from build123d import *

# Parameters (mm, degrees)
F0_W      = 57.15
F0_H      = 38.1
F1_DEPTH  = 58.42
F2_W      = 25.4
F2_H      = 25.4
F3_DEPTH  = 25.4
F4_W      = 50.8
F4_H      = 25.4
F5_DEPTH  = 50.8
F6_W      = 20.32
F6_H      = 20.32
F7_DEPTH  = 81.28
F8_W      = 22.86
F8_H      = 12.7
F9_DEPTH  = 25.4
F10_W     = 6.35
F10_H     = 6.35
F10_W_2   = 15.24
F10_H_2   = 5.08
F11_DEPTH = 12.7
F12_W     = 25.4
F12_H     = 9.817438
F13_DEPTH = 12.7
F14_W     = 19.21422
F14_H     = 50.8
F15_DEPTH = 6.35


with BuildPart() as f1:
    # F0 (on Top) → F1 (new body)
    with BuildSketch(Plane.XY):
        Rectangle(F0_W, F0_H)
    extrude(amount=F1_DEPTH)

    # F2 (on face) → F3 (join)
    with BuildSketch(Plane.XY.offset(58.42)):
        Rectangle(F2_W, F2_H)
    extrude(amount=F3_DEPTH)

    # F4 (on face) → F5 (cut)
    with BuildSketch(Plane.XY):
        Rectangle(F4_W, F4_H)
    extrude(amount=F5_DEPTH, mode=Mode.SUBTRACT)

    # F6 (on face) → F7 (cut)
    with BuildSketch(Plane.XY):
        Rectangle(F6_W, F6_H)
    extrude(amount=F7_DEPTH, mode=Mode.SUBTRACT)

    # F8 (on face) → F9 (cut)
    with BuildSketch(Plane(origin=(-28.575, 0, 0), x_dir=(0, -1, 0), z_dir=(-1, 0, 0))):
        with Locations((0, 31.75)):
            Rectangle(F8_W, F8_H)
    extrude(amount=-F9_DEPTH, mode=Mode.SUBTRACT)

    # F10 (on face) → F11 (cut)
    with BuildSketch(Plane(origin=(0, 12.7, 0), x_dir=(-1, 0, 0), z_dir=(0, 1, 0))):
        with Locations((-5.08, 74.295)):
            Rectangle(F10_W, F10_H)
        with Locations((5.08, 74.295)):
            Rectangle(F10_W, F10_H)
        with Locations((0, 63.942472)):
            Rectangle(F10_W_2, F10_H_2)
    extrude(amount=-F11_DEPTH, mode=Mode.SUBTRACT)

    # F12 (on face) → F13 (cut)
    with BuildSketch(Plane(origin=(0, 19.05, 0), x_dir=(-1, 0, 0), z_dir=(0, 1, 0))):
        with Locations((0, 15.411281)):
            Rectangle(F12_W, F12_H)
    extrude(amount=-F13_DEPTH, mode=Mode.SUBTRACT)

    # F14 (on face) → F15 (join)
    with BuildSketch(Plane.YZ.offset(28.575)):
        with Locations((0, 25.4)):
            Rectangle(F14_W, F14_H)
    extrude(amount=F15_DEPTH)


solid = f1.part
Design review of the part built by this model. Coordinates are the model's own, in mm. A direction names the side the tool comes from. Give positions to 0.01 mm unless a question says otherwise; leave off trailing zeros. Write each loop counter-clockwise with the first axis right and the second up, starting at its lowest first coordinate (ties: lowest second). Pieces come first, ordered by that corner, then holes. Notation, with made-up numbers: M 7.25,-25 L 60.25,-25 A8 cw 60.25,-15 Z; hole C 88.25,89 d6. An arc over 180 degrees is marked long. Answer as a JSON object with one key per item and string values. Group by question number.
1) Tool access review of faces 1 (the face through (-27, 0, 38.1)), 2 (the face through (12.7, 16, 15)), 3 (the face through (0, 12.7, 71)), 4 (the face through (0, 12.7, 25)): name each direction out of +Z, -Z, +X, -X, +Y, -Y from which nothing blocks a thin tool from reaching the whole face with its end or side.
2) Mouldability with a two-part tool opening along X and no side actions: class faces 5 (the face through (0, -12.7, 25)), 6 (the face through (-28.575, 0, 22)), 7 (the face through (-27, -11.43, 32)) as released by +X, released by -X, zero draft, split by the parting line, or undercut.
3) We need section A-A (y = 17). Give the boundary of the cut face in (x, z) (3 decimals).
4) Clearance check with flat-ended pins moving along their axes: pin 1 Ø1.3 at (y, z) = (12, 74) entering from -X; pin 2 Ø1.9 at (x, y) = (33, -1.5) entering from +Z; pin 3 Ø3 at (x, z) = (-2.5, 70) entering from -Y. State where each tip first meets the part, or that it passes through.
5) We need section D-D (x = 22). Give the boundary of the cut face in (y, z), and give its area (3 significant figures).
6) For line 1 along Y through (x, z) = (-16, 50); line 2 along X through (y, z) = (-3, 52) (3 decimals); line 3 along X through (y, z) = (10, 14) (3 decimals), list the stretches that pass through material, from the lowest coordinate up.
7) We need section B-B (y = -7.5). Give the boundary of the cut face in (x, z) (3 decimals).
8) We need section C-C (z = 47). Give the boundary of the cut face in (x, y) (3 decimals).
Answer key:
{
 "1": {"face 1": "-X", "face 2": "+Y", "face 3": "+Z, +X, -X, +Y", "face 4": "-Z"},
 "2": {"face 5": "undercut", "face 6": "released by -X", "face 7": "zero draft"},
 "3": {"outline": "M -28.575,0 L 28.575,0 L 28.575,58.42 L -28.575,58.42 Z; hole M -12.7,10.503 L 12.7,10.503 L 12.7,20.32 L -12.7,20.32 Z"},
 "4": {"pin 1": "stops at x = -12.7", "pin 2": "stops at z = 50.8", "pin 3": "stops at y = -12.7"},
 "5": {"outline": "M -19.05,0 L -12.7,0 L -12.7,50.8 L 12.7,50.8 L 12.7,0 L 19.05,0 L 19.05,58.42 L -19.05,58.42 Z", "area": "935 mm²"},
 "6": {"line 1": "y = -19.05 to -12.7, 12.7 to 19.05", "line 2": "x = -28.575 to -10.16, 10.16 to 28.575", "line 3": "x = -28.575 to -25.4, 25.4 to 28.575"},
 "7": {"outline": "M -28.575,0 L -25.4,0 L -25.4,25.4 L -28.575,25.4 Z; M -28.575,38.1 L -25.4,38.1 L -25.4,50.8 L -10.16,50.8 L -10.16,81.28 L 10.16,81.28 L 10.16,50.8 L 25.4,50.8 L 25.4,0 L 34.925,0 L 34.925,50.8 L 28.575,50.8 L 28.575,58.42 L 12.7,58.42 L 12.7,83.82 L -12.7,83.82 L -12.7,58.42 L -28.575,58.42 Z"},
 "8": {"outline": "M -28.575,-19.05 L 28.575,-19.05 L 28.575,-9.607 L 34.925,-9.607 L 34.925,9.607 L 28.575,9.607 L 28.575,19.05 L -28.575,19.05 Z; hole M -25.4,-12.7 L 25.4,-12.7 L 25.4,12.7 L -25.4,12.7 Z"}
}
